Autodesk Inventor part; units mm, degrees
ref_plane "YZ Plane" through (0, 0, 0) normal (1, 0, 0) x (0, 1, 0)
ref_plane "XZ Plane" through (0, 0, 0) normal (0, 1, 0) x (-1, 0, 0)
sketch "Эскиз1" plane through (0, 0, 0) normal (0, 1, 0) x (-1, 0, 0)
  circle A0 centre (0, 0) radius 3.95
  circle A1 centre (0, 0) radius 4.95
  line L0 (0, 0) -> (3.95, 2.9833)
  line L1 (0, 0) -> (3.95, -2.9833)
  point P0 (3.152, -2.3806)
  point P1 (3.152, 2.3806)
  dimension "d0" = 7.9
  dimension "d1" = 9.9
extrude "Выдавливание1" add sketch "Эскиз1" along normal blind 30 contours A0 L1 A1 L0 picked at (3.1693, 3.3115)
sketch "Эскиз2" plane through (0, 30, 0) normal (0, 1, 0) x (1, 0, 0)
  arc A0 (-3.152, -2.3806) -> (-4.0447, -1.8507) centre (-5.8533, -5.9145) ccw
  arc A1 (-4.0447, -1.8507) -> (-5.2016, -3.6565) centre (-4.4791, -2.8459) ccw
  line L0 (-5.2016, -3.6565) -> (-4.5303, -2.802)
  arc A2 (-3.9514, -2.9687) -> (-4.5303, -2.802) centre (-4.3197, -3.1592) ccw
  line L1 (0, 0) -> (-3.2711, 0)
  arc A3 (-4.0447, 1.8507) -> (-3.152, 2.3806) centre (-5.8533, 5.9145) ccw
  arc A4 (-5.2016, 3.6565) -> (-4.0447, 1.8507) centre (-4.4791, 2.8459) ccw
  line L2 (-5.2016, 3.6565) -> (-4.5303, 2.802)
  arc A5 (-4.5303, 2.802) -> (-3.9514, 2.9687) centre (-4.3197, 3.1592) ccw
  line L3 (-3.152, -2.3806) -> (-3.95, -2.9833)
  line L4 (-3.95, -2.9833) -> (-3.152, -2.3806)
  line L5 (-3.95, -2.9833) -> (-3.9514, -2.9687)
  line L6 (-3.152, 2.3806) -> (-3.95, 2.9833)
  line L7 (-3.95, 2.9833) -> (-3.9514, 2.9687)
extrude "Выдавливание2" add sketch "Эскиз2" against normal blind 30
sketch "Эскиз3" plane through (0, 30, 0) normal (0, 1, 0) x (1, 0, 0)
  arc A0 (-3.95, -2.9833) -> (-3.95, 2.9833) centre (0, 0) ccw
  line L0 (11.5, -6.95) -> (11.5, 6.95)
  arc A1 (-3.152, -2.3806) -> (-3.152, 2.3806) centre (0, 0) ccw
  arc A2 (0, -3.95) -> (0, 3.95) centre (0, 0) ccw
  line L1 (0, -4.95) -> (0, -3.95)
  line L2 (0, 3.95) -> (0, 4.95)
  line L3 (11.5, 6.95) -> (11.5, 10.95)
  line L4 (11.5, -6.95) -> (11.5, -10.95)
  line L5 (11.5, 10.95) -> (0, 10.95)
  line L6 (0, 10.95) -> (0, 4.95)
  line L7 (11.5, -10.95) -> (0, -10.95)
  line L8 (0, -10.95) -> (0, -4.95)
  dimension "d13" = 4
  dimension "d14" = 4
  dimension "d21" = 11.5
  dimension "d22" = 21.9
  dimension "d23" = 7
extrude "Выдавливание3" add sketch "Эскиз3" against normal blind 30 contours A0 L6 L5 L3 L0 L4 L7 L8
sketch "Эскиз4" plane through (11.5, 20, 4.95) normal (1, 0, 0) x (0, 0, -1)
  line L0 (4.95, -20) -> (4.95, 10)
  line L1 (1, 10) -> (8.9, 10)
  circle A0 centre (4.95, -12) radius 5
  line L2 (15.9, -20) -> (-6, -20)
  circle A1 centre (4.95, 2) radius 5
  line L3 (-6, 10) -> (15.9, 10)
  point P0 (7.3306, 10)
  point P1 (2.5694, 10)
  point P2 (4.95, -20)
  point P3 (4.95, 10)
  dimension "d15" = 10
  dimension "d16" = 8
  dimension "d17" = 10
  dimension "d18" = 8
extrude "Выдавливание4" cut sketch "Эскиз4" against normal blind 2
properties part number "крепление маркера 8мм"
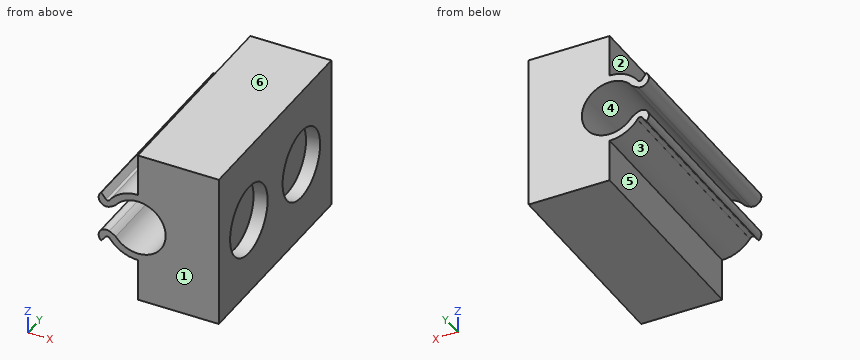
Design review of the part built by this model. Coordinates are the model's own, in mm. Face numbers are marked on the shaded views. A direction names the side the tool comes from. Round coordinates to 2 decimals unless told otherwise and drop trailing zeros. Write each loop counter-clockwise with the first axis right and the second up, starting at its lowest first coordinate (ties: lowest second). Pieces come first, ordered by that corner, then holes.
Item 1: For the marked faces 1 and 2, list the 3-axis set-ups (+Z, -Z, +X, -X, +Y, -Y) from which the entire face can be reached by the end or side of a thin tool; tool diameter is ignored.
Item 2: We need section D-D on x = -2.5. Write out the cut boundary in (y, z).
Item 3: We need section A-A on x = 1.5. Write out the cut boundary in (y, z).
Item 4: Clearance check with flat-ended pins moving along their axes: pin 1 Ø4 at (y, z) = (25, 7.5) entering from -X; pin 2 Ø5 at (y, z) = (10, -7) entering from -X; pin 3 Ø5 at (y, z) = (22, 0) entering from +X. State where each tip first meets the part, or that it passes through.
Item 5: For probe 1 along Y at (x, z) = (11, 0); probe 2 along Z at (x, y) = (11.15, 22); probe 3 along X at (y, z) = (5.5, 5.25), list the stretches that pass through material, from the lowest coordinate up.
Item 6: We need section B-B on z = 0. Write out the cut boundary in (x, y), and give its area (4 significant figures).
Item 7: The part is to be moulded in two halves that separate along Z. For the marked faces 3, 4, 5 and 6, say which applies: +Z half, -Z half, draft (parallel to the pull), parting line (faces both ways), or undercut.
Returned:
1. face 1: +Z, -Z, +X, -X, -Y
1. face 2: +Z, -X, +Y, -Y
2. outline: (0, -4.27) - (30, -4.27) - (30, -3.06) - (0, -3.06) - close; (0, 3.06) - (30, 3.06) - (30, 4.27) - (0, 4.27) - close
3. outline: (0, -10.95) - (30, -10.95) - (30, -3.65) - (0, -3.65) - close; (0, 3.65) - (30, 3.65) - (30, 10.95) - (0, 10.95) - close
4. pin 1: stops at x = 0
4. pin 2: stops at x = -2.06
4. pin 3: stops at x = 9.5
5. probe 1: y = 0 to 3, 13 to 17, 27 to 30
5. probe 2: z = -10.95 to -5, 5 to 10.95
5. probe 3: x = 0 to 11.5
6. outline: (3.95, 0) - (11.5, 0) - (11.5, 3) - (9.5, 3) - (9.5, 13) - (11.5, 13) - (11.5, 17) - (9.5, 17) - (9.5, 27) - (11.5, 27) - (11.5, 30) - (3.95, 30) - close
6. area: 186.5 mm2
7. face 3: -Z half
7. face 4: undercut
7. face 5: draft
7. face 6: +Z half
